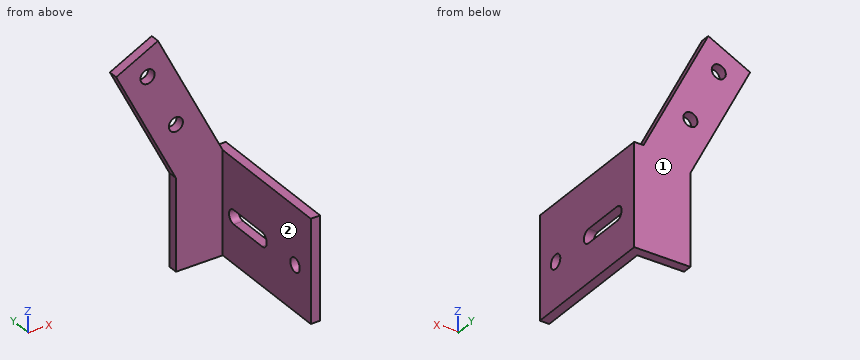
from build123d import *

# Parameters (mm, degrees)
SKETCH1_R           = 1.5
BOSS_EXTRUDE1_DEPTH = 2
SKETCH2_W           = 2
SKETCH2_H           = 21.888688708
BOSS_EXTRUDE2_DEPTH = 30
SKETCH4_R           = 1.5
CUT_EXTRUDE1_DEPTH  = 30


with BuildPart() as part:
    # Sketch1 → Boss-Extrude1 (new body)
    with BuildSketch(Plane(origin=(0, 0, 0), x_dir=(1, 0, 0), z_dir=(0, 1, 0))):
        Polygon((10.018564975, 30.6), (10.018564975, 8.711311292), (-3.787856503, -18.703932317), (-12.719216533, -14.206065265), (0.018564975, 11.087192922), (0.018564975, 30.6), align=None)
        with Locations(Location((0.018564975, -0.029187226, 0), (0, 0, 270))):
            Circle(SKETCH1_R, mode=Mode.SUBTRACT)
        with Locations(Location((-6.024680896, -12.029187226, 0), (0, 0, 270))):
            Circle(SKETCH1_R, mode=Mode.SUBTRACT)
    extrude(amount=BOSS_EXTRUDE1_DEPTH)

    # Sketch2 → Boss-Extrude2 (add)
    with BuildSketch(Plane(origin=(0, 2, 0), x_dir=(1, 0, 0), z_dir=(0, 1, 0))):
        with Locations((11.018564975, 19.655655646)):
            Rectangle(SKETCH2_W, SKETCH2_H)
    extrude(amount=-BOSS_EXTRUDE2_DEPTH)

    # Sketch4 → Cut-Extrude1 (cut)
    with BuildSketch(Plane(origin=(12.018564975, 0, 0), x_dir=(0, 0, -1), z_dir=(1, 0, 0))):
        with Locations((20.886224341, -23)):
            Circle(SKETCH4_R)
        with BuildLine():
            Line((22.386224341, -3.5), (22.386224341, -12.5))
            ThreePointArc((22.386224341, -12.5), (20.886224341, -14), (19.386224341, -12.5))
            Line((19.386224341, -12.5), (19.386224341, -3.5))
            ThreePointArc((19.386224341, -3.5), (20.886224341, -2), (22.386224341, -3.5))
        make_face()
    extrude(amount=-CUT_EXTRUDE1_DEPTH, mode=Mode.SUBTRACT)


solid = part.part
Here's how the part is built. I have some questions about the finished solid (model axes, mm). Face numbers are marked on the shaded views. A direction names the side the tool comes from. Round coordinates to 2 decimals unless told otherwise and drop trailing zeros. Write each loop counter-clockwise with the first axis right and the second up, starting at its lowest first coordinate (ties: lowest second). Pieces come first, ordered by that corner, then holes. Notation, with made-up numbers: (59, 36.5) -> (87, 36.5) arc R11 cw to (87, 41.5) -> close; hole circle Ø9 at (-0.5, -36.5). An arc over 180 degrees is marked (long way). One line per item, written item: value.
1) Suppose I cut it at A-A on y = -10. List the corners of the cut face in (x, z) for me, plus the area to 3 significant figures.
Filled sheet:
outline: (10.02, -30.6) -> (12.02, -30.6) -> (12.02, -22.39) -> (10.02, -22.39) -> close; (10.02, -19.39) -> (12.02, -19.39) -> (12.02, -8.71) -> (10.02, -8.71) -> close
area: 37.8 mm2
2) If I drill on line 1 (Z direction, x = 10.25, y = -8.5); line 2 (Y direction, x = 1, z = -13.5); line 3 (X direction, y = -1.25, z = -28), over which ranges is the centre line in solid material (lowest first)? Write a range as [from, to].
Filled sheet:
line 1: z = [-30.6, -22.39], [-19.39, -8.71]
line 2: y = [0, 2]
line 3: x = [10.02, 12.02]
3) Suppose I cut it at B-B on z = -17. List the corners of the cut face in (x, y) for me.
Filled sheet:
outline: (0.02, 0) -> (10.02, 0) -> (10.02, -28) -> (12.02, -28) -> (12.02, 2) -> (0.02, 2) -> close
4) I'm going to push flat-ended pins straight in: pin 1 Ø1.5 at (y, z) = (-2, -2) entering from -X; pin 2 Ø6 at (y, z) = (-10.5, -8) entering from -X; pin 3 Ø0.6 at (x, y) = (10.5, -13) entering from +Z; pin 4 Ø2 at (y, z) = (1, -17.5) entering from -X. Where does each tip first touch, or does it pass through?
Filled sheet:
pin 1: passes through
pin 2: stops at x = 10.02
pin 3: stops at z = -8.71
pin 4: stops at x = 0.02
5) Suppose I cut it at D-D on z = -2. List the corners of the cut face in (x, y) for me.
Filled sheet:
outline: (-4.56, 0) -> (6.64, 0) -> (6.64, 2) -> (-4.56, 2) -> close
6) Suppose I cut it at C-C on x = -9.5. List the corners of the cut face in (y, z) for me.
Filled sheet:
outline: (0, 7.81) -> (2, 7.81) -> (2, 15.83) -> (0, 15.83) -> close
7) For the marked faces 1 and 2, which set-ups out of +Z, -Z, +X, -X, +Y, -Y let a thin tool reach every point of the face, with its end or its side?
Filled sheet:
face 1: +Z, -Z, +X, -X, +Y
face 2: +Z, -Z, -X, -Y
